For this review, use the dimensioned drawing (mm, ordinates from the lowest corner) and the shaded views. Coordinates: 2 decimals unless noted, no trailing zeros. Loops run counter-clockwise (first coordinate to the right, second up) from the corner with the lowest first, then second, coordinate; pieces in that order, holes last. Notation, with made-up numbers: (27, -17.5) - (47, -17.5) arc R32 ccw to (47, 19.5) - close; hole circle Ø9 at (42.5, -2). An arc over 180 degrees is marked (long way). Answer in a Markdown table with one row per item. Add a question column.
(1) We need section B-B on x = 12. Write out the cut boundary in (y, z).
(2) We need section D-D on x = 3.5. Write out the cut boundary in (y, z).
(3) Mouldability with a two-part tool opening along X and no side actions: class the marked faces 1, 2, 3 and 4 as +X half, -X half, draft (parallel to the pull), parting line (faces both ways), or undercut.
(4) For P1, Ø0.8, axis at y = 9.5, z = 4, coming from the -X side; P2, Ø0.8, axis at y = 1.5, z = 0.5, coming from the -X side; P3, Ø3, axis at x = 4, y = 5, coming from the +Z side; P4, Ø1.5, axis at x = 10.5, z = 2.5, coming from the +Y side, all flat-tipped, find the tip position at first contact; note any pin that passes through.
(5) For line 1 along Y through (x, z) = (4, 3.4); line 2 along X through (y, z) = (5.25, 2.1); line 3 along X through (y, z) = (4, 4.65), list the stretches that pass through material, from the lowest coordinate up.
(6) We need section C-C on y = 4.25. Write out the cut boundary in (x, z).
(7) We need section A-A on z = 2.75. Write out the cut boundary in (x, y), plus the area to 3 significant figures.
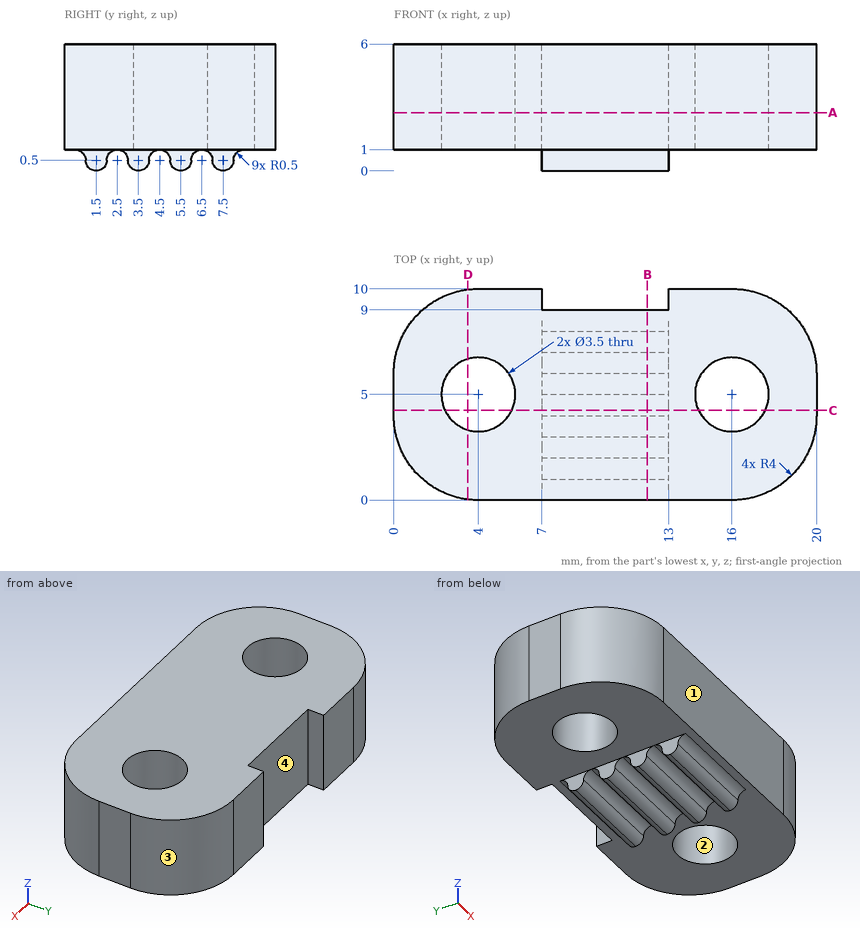
Outcome:
| question | item | result |
|---|---|---|
| 1 | outline | (0, 1) - (0.5, 1) arc R0.5 cw to (1, 0.5) arc R0.5 ccw to (2, 0.5) arc R0.5 cw to (3, 0.5) arc R0.5 ccw to (4, 0.5) arc R0.5 cw to (5, 0.5) arc R0.5 ccw to (6, 0.5) arc R0.5 cw to (7, 0.5) arc R0.5 ccw to (8, 0.5) arc R0.5 cw to (8.5, 1) - (9, 1) - (9, 6) - (0, 6) - close |
| 2 | outline | (0.03, 1) - (3.32, 1) - (3.32, 6) - (0.03, 6) - close; (6.68, 1) - (9.97, 1) - (9.97, 6) - (6.68, 6) - close |
| 3 | face 1 | draft |
| 3 | face 2 | undercut |
| 3 | face 3 | +X half |
| 3 | face 4 | undercut |
| 4 | P1 | x = 1.47 |
| 4 | P2 | x = 7 |
| 4 | P3 | through |
| 4 | P4 | y = 9 |
| 5 | line 1 | 0 to 3.25, 6.75 to 10 |
| 5 | line 2 | 0 to 2.27, 5.73 to 14.27, 17.73 to 20 |
| 5 | line 3 | 0 to 2.56, 5.44 to 14.56, 17.44 to 20 |
| 6 | outline | (0, 1) - (2.42, 1) - (2.42, 6) - (0, 6) - close; (5.58, 1) - (7, 1) - (7, 0.93) - (13, 0.93) - (13, 1) - (14.42, 1) - (14.42, 6) - (5.58, 6) - close; (17.58, 1) - (20, 1) - (20, 6) - (17.58, 6) - close |
| 7 | outline | (0, 4) arc R4 ccw to (4, 0) - (16, 0) arc R4 ccw to (20, 4) - (20, 6) arc R4 ccw to (16, 10) - (13, 10) - (13, 9) - (7, 9) - (7, 10) - (4, 10) arc R4 ccw to (0, 6) - close; hole circle Ø3.5 at (4, 5); hole circle Ø3.5 at (16, 5) |
| 7 | area | 161 mm² |
